Study the drawing (mm; zero at the part's minimum x, y, z) and answer. A direction names the side the tool comes from. Give positions to 0.01 mm unless a question says otherwise; leave off trailing zeros. Order: outer loops, then holes, each group sorted by start corner. A loop starts at its lowest first (then second) coordinate and runs counter-clockwise, first axis right, second up. Notation, with made-up numbers: (55, 53.25) -> (89, 53.25) arc R18 cw to (89, 69.25) -> close; hole circle Ø1 at (72, 39). An arc over 180 degrees is marked (long way). Answer as CSV lines item,"result". Start each with the question number.
1. Find the intervals of material crossed by L1, parallel to Z at x = 25, y = 0.9; L2, parallel to Z at x = 26.5, y = 5; L3, parallel to X at y = 1.15, z = 25, in increasing order.
2. A cutting plane is placed at B-B (x = 25). Give the vertices of the cut face in (y, z), then the cut area to 3 significant figures.
3. For the marked faces 4 and 5, determine the directions among +Z, -Z, +X, -X, +Y, -Y from which every point of the face is accessible in a straight line to the end or side of a thin tool.
4. Flat-ended cylindrical pins translate along their axes: pin 1 (2 mm diameter, centred on x = 17.5, z = 8.5, fed in from -Y); pin 2 (7.5 mm diameter, centred on x = 25, z = 25, fed in from +Y); pin 3 (3 mm diameter, centred on y = 5, z = 26.5, fed in from -X). Find the tip coordinate at first contact, or state that the pin passes through.
5. A cutting plane is placed at D-D (z = 6.5). Give the vertices of the cut face in (x, y), then the cut area to 3 significant figures.
6. A cutting plane is placed at A-A (y = 3.5). Give the vertices of the cut face in (x, z), then the cut area to 3 significant figures.
7. For a pull along X with two mould halves and no side action, classify the marked faces 1, 2 and 3 as released by +X, released by -X, zero draft, split by the parting line, or undercut.
8. A cutting plane is placed at C-C (z = 25). Give the vertices of the cut face in (x, y).
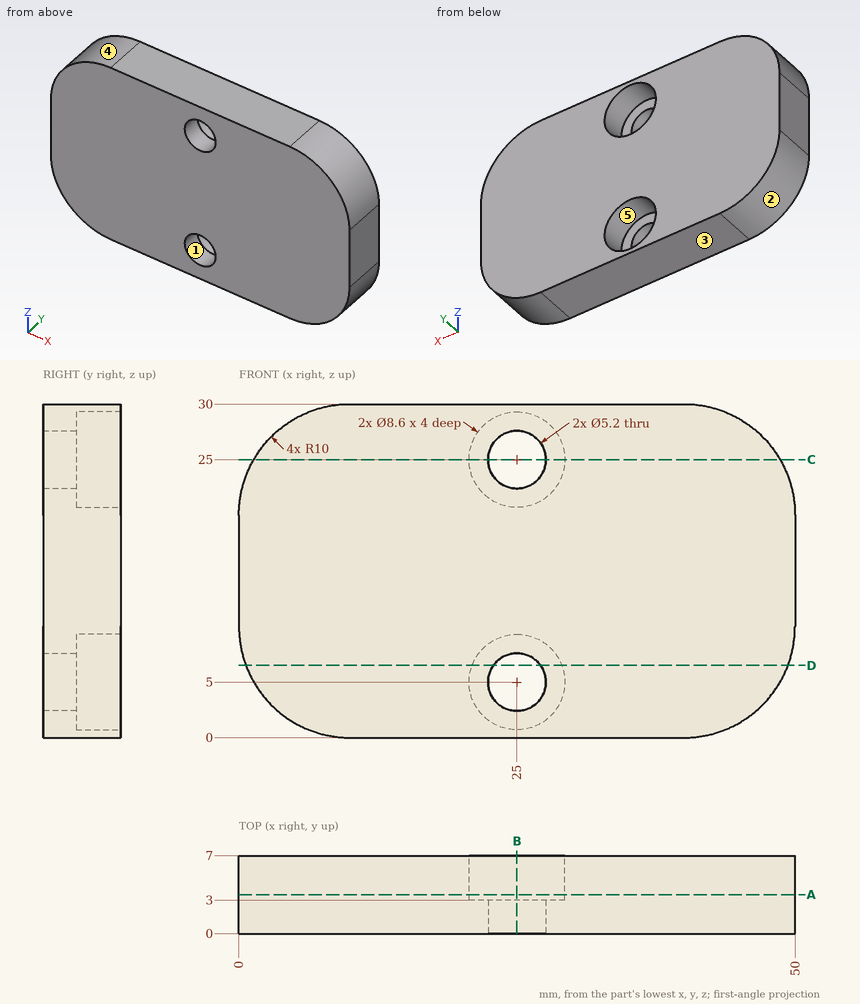
Answer sheet:
1,L1,"z = 0 to 2.4, 7.6 to 22.4, 27.6 to 30"
1,L2,"z = 0 to 0.97, 9.03 to 20.97, 29.03 to 30"
1,L3,"x = 1.34 to 22.4, 27.6 to 48.66"
2,outline,"(0, 0) -> (7, 0) -> (7, 0.7) -> (3, 0.7) -> (3, 2.4) -> (0, 2.4) -> close; (0, 7.6) -> (3, 7.6) -> (3, 9.3) -> (7, 9.3) -> (7, 20.7) -> (3, 20.7) -> (3, 22.4) -> (0, 22.4) -> close; (0, 27.6) -> (3, 27.6) -> (3, 29.3) -> (7, 29.3) -> (7, 30) -> (0, 30) -> close"
2,area,"110 mm^2"
3,face 4,"+Z, -X, +Y, -Y"
3,face 5,"+Y"
4,pin 1,"stops at y = 0"
4,pin 2,"stops at y = 3"
4,pin 3,"stops at x = 1.34"
5,outline,"(0.63, 0) -> (22.88, 0) -> (22.88, 3) -> (20.97, 3) -> (20.97, 7) -> (0.63, 7) -> close; (27.12, 0) -> (49.37, 0) -> (49.37, 7) -> (29.03, 7) -> (29.03, 3) -> (27.12, 3) -> close"
5,area,"296 mm^2"
6,outline,"(0, 10) arc R10 ccw to (10, 0) -> (40, 0) arc R10 ccw to (50, 10) -> (50, 20) arc R10 ccw to (40, 30) -> (10, 30) arc R10 ccw to (0, 20) -> close; hole circle Ø8.6 at (25, 5); hole circle Ø8.6 at (25, 25)"
6,area,"1,300 mm^2"
7,face 1,"undercut"
7,face 2,"released by -X"
7,face 3,"zero draft"
8,outline,"(1.34, 0) -> (22.4, 0) -> (22.4, 3) -> (20.7, 3) -> (20.7, 7) -> (1.34, 7) -> close; (27.6, 0) -> (48.66, 0) -> (48.66, 7) -> (29.3, 7) -> (29.3, 3) -> (27.6, 3) -> close"
